Could you check a few things on this model? Use its own coordinates, in mm. Round coordinates to 2 decimals unless told otherwise and drop trailing zeros. Write each loop counter-clockwise with the first axis right and the second up, starting at its lowest first coordinate (ties: lowest second). Pieces come first, ordered by that corner, then holes. Notation, with made-up numbers: (80, 44.25) -> (85, 44.25) arc R35 ccw to (85, 79.25) -> close; hole circle Ø2 at (81.5, -38.5). An arc over 180 degrees is marked (long way). One line per question, with ' | ' between items. Start each with the question number.
1. For pin 1 Ø8 at (x, y) = (18, -47.5) entering from -Z, with a flat end and sliding along its axis, tell me the tip position at first contact or that it passes through.
2. If I drill on line 1 along Z through (x, y) = (18.5, -53.5); line 2 along Z through (x, y) = (19.05, -37); line 3 along X through (y, z) = (-35.5, 355.6), over which ranges is the centre line in solid material (lowest first)? Write a range as [from, to].
3. Imagine slicing it at B-B, the plane z = 355.6. List the corners of the cut face in (x, y) for me.
4. Imagine slicing it at A-A, the plane x = 19.05. List the corners of the cut face in (y, z) for me, and give its area (3 significant figures).
5. Imagine slicing it at C-C, the plane y = -49. List the corners of the cut face in (x, z) for me.
from build123d import *

# Parameters (mm, degrees)
SKETCH1_W           = 19.05
SKETCH1_H           = 76.2
REVOLVE1_ANGLE      = 180
SKETCH2_W           = 38.1
SKETCH2_H           = 76.2
BOSS_EXTRUDE1_DEPTH = 381
SKETCH3_R           = 3.9878
CUT_EXTRUDE1_DEPTH  = 391.408824183
SKETCH4_R           = 3.9878
CUT_EXTRUDE2_DEPTH  = 391.408824183


with BuildPart() as part:
    # Sketch1 → Revolve1 (revolve)
    with BuildSketch(Plane.XY):
        with Locations((9.525, -38.1)):
            Rectangle(SKETCH1_W, SKETCH1_H)
    revolve(axis=Axis((19.05, 0, 0), (0, -1, 0)), revolution_arc=REVOLVE1_ANGLE)

    # Sketch2 → Boss-Extrude1 (add)
    with BuildSketch(Plane.XY):
        with Locations((19.05, -38.1)):
            Rectangle(SKETCH2_W, SKETCH2_H)
    extrude(amount=BOSS_EXTRUDE1_DEPTH)

    # Sketch3 → Cut-Extrude1 (cut, through all)
    with BuildSketch(Plane(origin=(0, 0, 0), x_dir=(1, 0, 0), z_dir=(0, 1, 0))):
        with Locations(Location((19.05, 0, 0), (0, 0, 180))):
            Circle(SKETCH3_R)
    extrude(amount=-CUT_EXTRUDE1_DEPTH, mode=Mode.SUBTRACT)

    # Sketch4 → Cut-Extrude2 (cut, through all)
    with BuildSketch(Plane(origin=(0, 0, 0), x_dir=(1, 0, 0), z_dir=(0, 1, 0))):
        with Locations(Location((19.05, -355.6, 0), (0, 0, 180))):
            Circle(SKETCH4_R)
    extrude(amount=-CUT_EXTRUDE2_DEPTH, mode=Mode.SUBTRACT)


solid = part.part
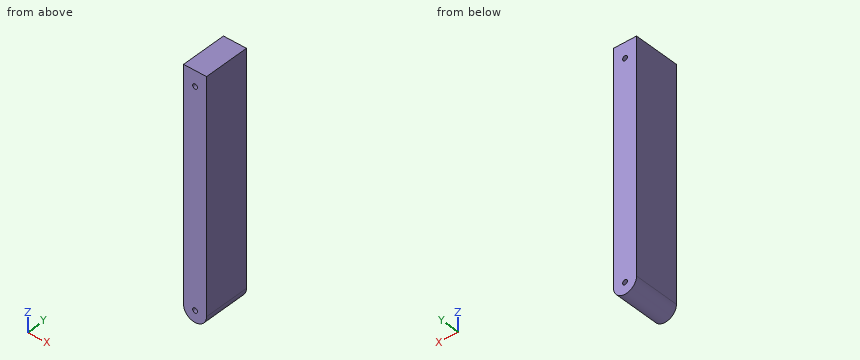
Geometry results:
1) pin 1: stops at z = -19.05
2) line 1: z = [-19.04, -3.95], [3.95, 351.65], [359.55, 381] | line 2: z = [-19.05, -3.99], [3.99, 351.61], [359.59, 381] | line 3: x = [0, 15.06], [23.04, 38.1]
3) outline: (0, -76.2) -> (15.06, -76.2) -> (15.06, 0) -> (0, 0) -> close; (23.04, -76.2) -> (38.1, -76.2) -> (38.1, 0) -> (23.04, 0) -> close
4) outline: (-76.2, -19.05) -> (0, -19.05) -> (0, -3.99) -> (-76.2, -3.99) -> close; (-76.2, 3.99) -> (0, 3.99) -> (0, 351.61) -> (-76.2, 351.61) -> close; (-76.2, 359.59) -> (0, 359.59) -> (0, 381) -> (-76.2, 381) -> close | area: 29,300 mm2
5) outline: (0, 0) arc R19.05 ccw to (38.1, 0) -> (38.1, 381) -> (0, 381) -> close; hole circle Ø7.98 at (19.05, 0); hole circle Ø7.98 at (19.05, 355.6)
